Autodesk Inventor part; units mm, degrees
ref_plane "YZ Plane" through (0, 0, 0) normal (1, 0, 0) x (0, 1, 0)
ref_plane "XZ Plane" through (0, 0, 0) normal (0, 1, 0) x (-1, 0, 0)
ref_plane "XY Plane" through (0, 0, 0) normal (0, 0, 1) x (1, 0, 0)
sketch "Sketch1" plane through (0, 0, 0) normal (0, 0, 1) x (1, 0, 0)
  line L0 (0, 0) -> (-10, 0)
  line L1 (-10, 0) -> (-10, 45)
  line L2 (-10, 45) -> (0, 45)
  line L3 (0, 45) -> (0, 0)
  dimension "d0" = 10
  dimension "d1" = 45
extrude "Extrusion1" add sketch "Sketch1" along normal blind 5
sketch "Sketch2" plane through (0, 0, 5) normal (0, 0, 1) x (1, 0, 0)
  line L0 (0, 0) -> (0, 45)
  line L1 (-10, 45) -> (-10, 0)
  line L2 (0, 45) -> (-10, 45)
  line L3 (-10, 0) -> (0, 0)
  point P0 (-5, 37.5)
  point P1 (-5, 7.5)
  dimension "d4" = 5
  dimension "d5" = 5
  dimension "d6" = 7.5
  dimension "d7" = 7.5
  dimension "d8" = 30
hole "Hole1" at (-5, 37.5, 5) at (-5, 7.5, 5) direction (0, 0, -1) diameter 4.5 end through all countersink diameter 9.4 countersink angle 90
properties part number "Pancake_Side Piece Short 2" material "Wood (Birch)"
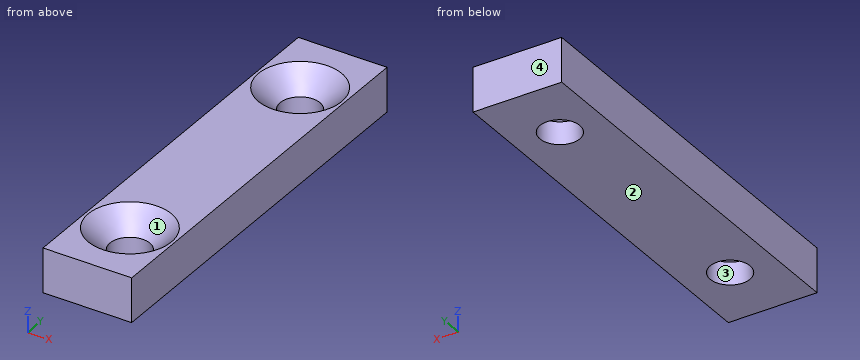
The model under review builds one solid part; all positions refer to its coordinate system, in mm. Face numbers are marked on the shaded views. Coordinates: 2 decimals unless noted, no trailing zeros. Loops run counter-clockwise (first coordinate to the right, second up) from the corner with the lowest first, then second, coordinate; pieces in that order, holes last. Notation, with made-up numbers: M 72.5,40 L 127.5,40 A21 cw 127.5,46 Z; hole C 69.25,87.5 d1. An arc over 180 degrees is marked long. Put each result on its own line as item: value. Start each with the question number.
Q1. Add section A-A (y = 37.5). Write out the cut boundary in (x, z).
Q2. Clearance check with flat-ended pins moving along their axes: pin 1 (4 mm diameter, centred on x = -5, y = 37.5, fed in from -Z); pin 2 (3 mm diameter, centred on x = -7, y = 8, fed in from +Z). State where each tip first meets the part, or that it passes through.
Q3. Add section B-B (x = -5). Write out the cut boundary in (y, z).
Q4. Wall thickness on line 1 (Y direction, x = -5, z = 1.25); line 2 (X direction, y = 37.5, z = 1); line 3 (Y direction, x = -3.75, z = 0.8): over which ranges is each line inside the solid? List them lowest first.
Q5. Add section C-C (z = 1.85). Write out the cut boundary in (x, y), and give its area (3 significant figures).
Q6. Add section D-D (z = 3.6). Write out the cut boundary in (x, y), and give its area (3 significant figures).
Q7. The part is to be moulded in two halves that separate along Y. For the marked faces 1, 2, 3 and 4, say which applies: +Y half, -Y half, draft (parallel to the pull), parting line (faces both ways), or undercut.
Answers:
1. outline: M -10,0 L -7.25,0 L -7.25,2.55 L -9.7,5 L -10,5 Z; M -2.75,0 L 0,0 L 0,5 L -0.3,5 L -2.75,2.55 Z
2. pin 1: passes through
2. pin 2: stops at z = 3.86
3. outline: M 0,0 L 5.25,0 L 5.25,2.55 L 2.8,5 L 0,5 Z; M 9.75,0 L 35.25,0 L 35.25,2.55 L 32.8,5 L 12.2,5 L 9.75,2.55 Z; M 39.75,0 L 45,0 L 45,5 L 42.2,5 L 39.75,2.55 Z
4. line 1: y = 0 to 5.25, 9.75 to 35.25, 39.75 to 45
4. line 2: x = -10 to -7.25, -2.75 to 0
4. line 3: y = 0 to 5.63, 9.37 to 35.63, 39.37 to 45
5. outline: M -10,0 L 0,0 L 0,45 L -10,45 Z; hole C -5,7.5 d4.5; hole C -5,37.5 d4.5
5. area: 418 mm^2
6. outline: M -10,0 L 0,0 L 0,45 L -10,45 Z; hole C -5,7.5 d6.6; hole C -5,37.5 d6.6
6. area: 382 mm^2
7. face 1: undercut
7. face 2: draft
7. face 3: undercut
7. face 4: +Y half
